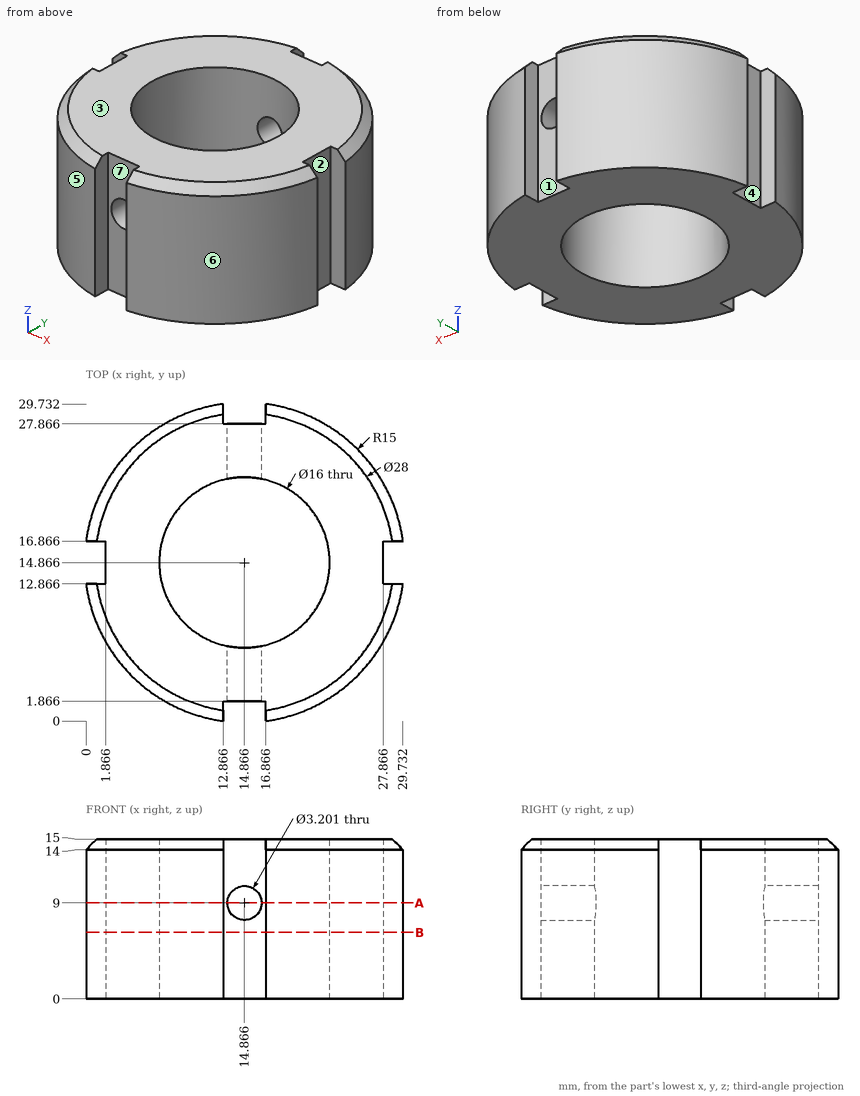
The drawing under review shows one solid part. Ordinate dimensions are in mm from its lowest x, y, z. A direction names the side the tool comes from. Give positions to 0.01 mm unless a question says otherwise; leave off trailing zeros. Write each loop counter-clockwise with the first axis right and the second up, starting at its lowest first coordinate (ties: lowest second). Pieces come first, ordered by that corner, then holes. Notation, with made-up numbers: (5.25, -22.5) - (51.25, -22.5) arc R25 ccw to (51.25, -6.5) - close; hole circle Ø1 at (-25, -27.5). An arc over 180 degrees is marked (long way). Answer in a Markdown table with one row per item. Add a question column.
1. Tool access review of the marked faces 1, 2, 3 and 4: name each direction out of +Z, -Z, +X, -X, +Y, -Y from which nothing blocks a thin tool from reaching the whole face with its end or side.
2. Insertion check: P1, Ø0.9, axis at x = 28.5, z = 5, coming from the +Y side; P2, Ø1, axis at x = 13.5, z = 6, coming from the -Y side; P3, Ø9.5, axis at x = 14.87, y = 14.87, coming from the -Z side; P4, Ø2, axis at y = 0.5, z = 8, coming from the +X side. Each pin has a flat end and moves straight along its axis. Give the tip position at first contact, or say it passes through.
3. We need section A-A on z = 9. Write out the cut boundary in (x, y), then the cut area to 3 significant figures.
4. Draft analysis for pull direction X (two halves, no side actions). For the marked faces 5, 6 and 7, state which applies: +X half, -X half, draft (parallel to the pull), parting line (faces both ways), or undercut.
5. Wall thickness on line 1 along Y through (x, z) = (10, 2.25) (1 decimal); line 2 along X through (y, z) = (4.8, 9) (1 decimal); line 3 along Y through (x, z) = (13.25, 4.75): over which ranges is each line inside the solid? List them lowest first. Write a range as [from, to].
6. We need section B-B on z = 6.25. Write out the cut boundary in (x, y).
Ans:
| question | item | result |
|---|---|---|
| 1 | face 1 | +Z, -Z, +Y |
| 1 | face 2 | +Z, -Z, +X |
| 1 | face 3 | +Z, +X, -X, +Y, -Y |
| 1 | face 4 | +Z, -Z, -X |
| 2 | P1 | stops at y = 22.02 |
| 2 | P2 | stops at y = 1.87 |
| 2 | P3 | passes through |
| 2 | P4 | stops at x = 21.67 |
| 3 | outline | (0, 12.87) arc R15 ccw to (12.87, 0) - (12.87, 1.87) - (13.27, 1.87) - (13.27, 7.03) arc R8 cw to (13.27, 22.7) - (13.27, 27.87) - (12.87, 27.87) - (12.87, 29.73) arc R15 ccw to (0, 16.87) - (1.87, 16.87) - (1.87, 12.87) - close; (16.47, 1.87) - (16.87, 1.87) - (16.87, 0) arc R15 ccw to (29.73, 12.87) - (27.87, 12.87) - (27.87, 16.87) - (29.73, 16.87) arc R15 ccw to (16.87, 29.73) - (16.87, 27.87) - (16.47, 27.87) - (16.47, 22.7) arc R8 cw to (16.47, 7.03) - close |
| 3 | area | 442 mm^2 |
| 4 | face 5 | -X half |
| 4 | face 6 | +X half |
| 4 | face 7 | undercut |
| 5 | line 1 | y = [0.7, 8.5], [21.2, 29.1] |
| 5 | line 2 | x = [3.7, 13.3], [16.5, 26] |
| 5 | line 3 | y = [1.87, 7.03], [22.7, 27.87] |
| 6 | outline | (0, 12.87) arc R15 ccw to (12.87, 0) - (12.87, 1.87) - (16.87, 1.87) - (16.87, 0) arc R15 ccw to (29.73, 12.87) - (27.87, 12.87) - (27.87, 16.87) - (29.73, 16.87) arc R15 ccw to (16.87, 29.73) - (16.87, 27.87) - (12.87, 27.87) - (12.87, 29.73) arc R15 ccw to (0, 16.87) - (1.87, 16.87) - (1.87, 12.87) - close; hole circle Ø16 at (14.87, 14.87) |
